Model file for the job. Use its own axes, mm. Coordinates: 2 decimals unless noted, no trailing zeros. Loops run counter-clockwise (first coordinate to the right, second up) from the corner with the lowest first, then second, coordinate; pieces in that order, holes last. Notation, with made-up numbers: (-38.75, -28) -> (-8.75, -28) arc R26 cw to (-8.75, 6) -> close; hole circle Ø9 at (43.25, 17). An arc over 180 degrees is marked (long way). Use one line per item in the form item = value.
```python
from build123d import *

# Parameters (mm, degrees)
ESBO_O1_R                = 2
ESBO_O1_W                = 20
ESBO_O1_H                = 20
RESSALTO_EXTRUS_O1_DEPTH = 10
ESBO_O3_R                = 4.5
CORTE_EXTRUS_O1_DEPTH    = 4


with BuildPart() as part:
    # Esboço1 → Ressalto-extrusão1 (new body)
    with BuildSketch(Plane.XY):
        with BuildLine():
            Line((107, 94.817541634), (50, 0))
            Line((50, 0), (107, -94.817541634))
            ThreePointArc((107, -94.817541634), (111.571067812, -111.571067812), (94.817541634, -107))
            Line((94.817541634, -107), (0, -50))
            Line((0, -50), (-94.817541634, -107))
            ThreePointArc((-94.817541634, -107), (-111.571067812, -111.571067812), (-107, -94.817541634))
            Line((-107, -94.817541634), (-50, 0))
            Line((-50, 0), (-107, 94.817541634))
            ThreePointArc((-107, 94.817541634), (-111.571067812, 111.571067812), (-94.817541634, 107))
            Line((-94.817541634, 107), (0, 50))
            Line((0, 50), (94.817541634, 107))
            ThreePointArc((94.817541634, 107), (111.571067812, 111.571067812), (107, 94.817541634))
        make_face()
        with Locations((-104.5, 104.5)):
            Circle(ESBO_O1_R, mode=Mode.SUBTRACT)
        with Locations((104.5, 104.5)):
            Circle(ESBO_O1_R, mode=Mode.SUBTRACT)
        with Locations((104.5, -104.5)):
            Circle(ESBO_O1_R, mode=Mode.SUBTRACT)
        with Locations((-104.5, -104.5)):
            Circle(ESBO_O1_R, mode=Mode.SUBTRACT)
        with Locations((25, -25)):
            Rectangle(ESBO_O1_W, ESBO_O1_H, mode=Mode.SUBTRACT)
        with Locations((25, 25)):
            Rectangle(ESBO_O1_W, ESBO_O1_H, mode=Mode.SUBTRACT)
        with Locations((-25, 25)):
            Rectangle(ESBO_O1_W, ESBO_O1_H, mode=Mode.SUBTRACT)
        with Locations((-25, -25)):
            Rectangle(ESBO_O1_W, ESBO_O1_H, mode=Mode.SUBTRACT)
    extrude(amount=RESSALTO_EXTRUS_O1_DEPTH)

    # Esboço3 → Corte-extrusão1 (cut)
    with BuildSketch(Plane(origin=(0, 0, 0), x_dir=(-1, 0, 0), z_dir=(0, 0, -1))):
        with Locations((-104.5, 104.5)):
            Circle(ESBO_O3_R)
        with Locations((104.5, 104.5)):
            Circle(ESBO_O3_R)
        with Locations((104.5, -104.5)):
            Circle(ESBO_O3_R)
        with Locations((-104.5, -104.5)):
            Circle(ESBO_O3_R)
    extrude(amount=-CORTE_EXTRUS_O1_DEPTH, mode=Mode.SUBTRACT)


solid = part.part
```
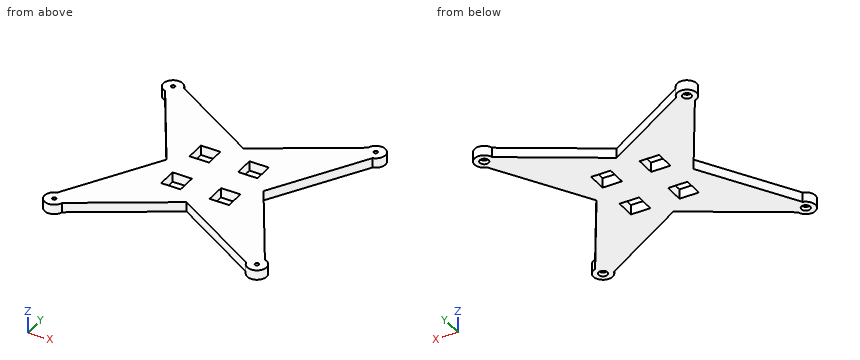
Q1. Band-saw the part on C-C, the plane x = 76. Write the cut outline in (y, z).
Result:
outline = (-95.69, 0) -> (-43.25, 0) -> (-43.25, 10) -> (-95.69, 10) -> close; (43.25, 0) -> (95.69, 0) -> (95.69, 10) -> (43.25, 10) -> close
Q2. Band-saw the part on A-A, the plane y = 87.5. Write the cut outline in (x, z), and give its area (3 significant figures).
Result:
outline = (-102.6, 0) -> (-62.38, 0) -> (-62.38, 10) -> (-102.6, 10) -> close; (62.38, 0) -> (102.6, 0) -> (102.6, 10) -> (62.38, 10) -> close
area = 804 mm2
Q3. Pin check, flat tips, straight feed: pin 1 Ø7 at (x, y) = (-105.5, 104) entering from -Z; pin 2 Ø4.5 at (x, y) = (104.5, 105) entering from -Z; pin 3 Ø4 at (x, z) = (4, 7.5) entering from +Y; pin 4 Ø3 at (x, z) = (-23, 7) entering from -Y. Stop position of each tip, or through.
Result:
pin_1 = 0
pin_2 = 4
pin_3 = 53.61
pin_4 = -64.73
Q4. Band-saw the part on D-D, the plane y = 30. Write the cut outline in (x, z), and give its area (3 significant figures).
Result:
outline = (-68.03, 0) -> (-35, 0) -> (-35, 10) -> (-68.03, 10) -> close; (-15, 0) -> (15, 0) -> (15, 10) -> (-15, 10) -> close; (35, 0) -> (68.03, 0) -> (68.03, 10) -> (35, 10) -> close
area = 961 mm2
Q5. Band-saw the part on B-B, the plane z = 2.5. State how many separate pieces and enclosed holes the cut face has, and give its area (3 significant figures).
Result:
separate_pieces = 1
enclosed_holes = 8
area = 23,000 mm2
Q6. Wall check: line 1 along X through (y, z) = (-24.5, 4.5); line 2 along Y through (x, z) = (-104.5, 3.15); line 3 along X through (y, z) = (-104.5, 6.5). Give the ranges that are in metal, low to high.
Result:
line_1 = -64.73 to -35, -15 to 15, 35 to 64.73
line_2 = -114.5 to -109, -100 to -90.66, 90.66 to 100, 109 to 114.5
line_3 = -114.5 to -106.5, -102.5 to -90.66, 90.66 to 102.5, 106.5 to 114.5
